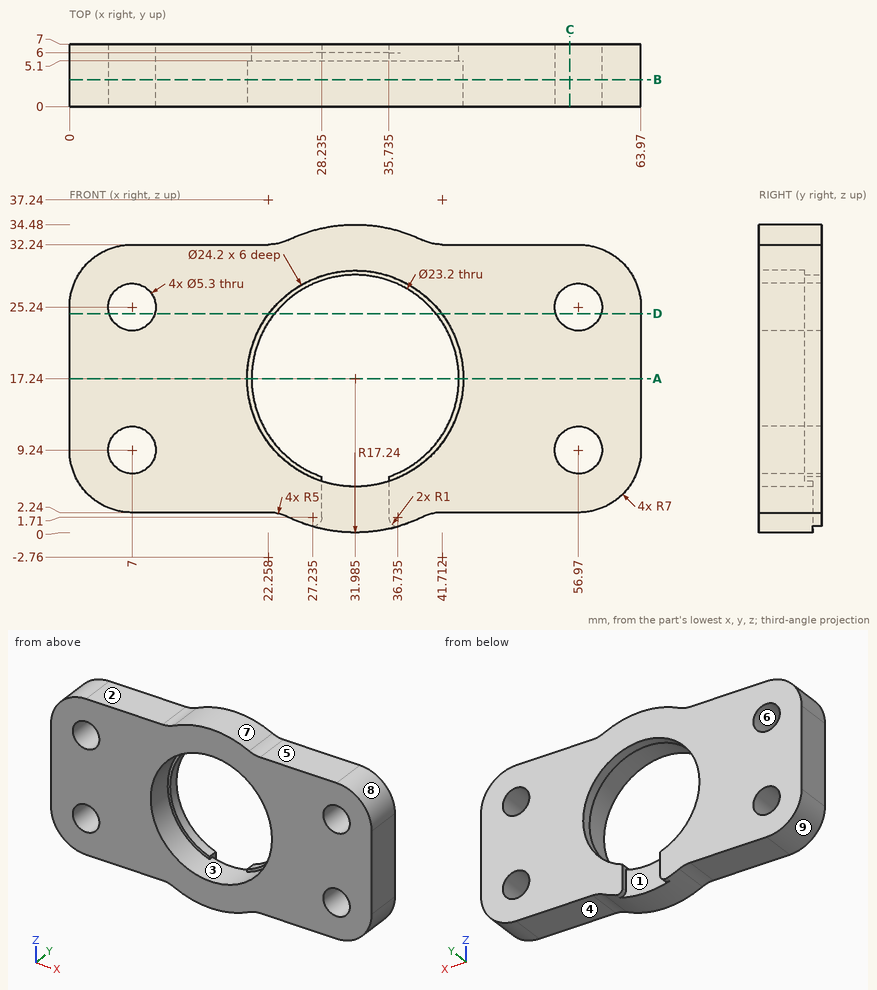
Study the drawing (mm; zero at the part's minimum x, y, z) and answer. A direction names the side the tool comes from. Coordinates: 2 decimals unless noted, no trailing zeros. Write each loop counter-clockwise with the first axis right and the second up, starting at its lowest first coordinate (ties: lowest second). Pieces come first, ordered by that corner, then holes. Notation, with made-up numbers: (33.25, 19) - (64.25, 19) arc R14 cw to (64.25, 40) - close; hole circle Ø6 at (-23.75, -35.5). An arc over 180 degrees is marked (long way). Answer as a JSON object with one key per item and string values.
Q1. For a pull along X with two mould halves and no side action, classify the marked faces 6, 7, 8 and 9 as pulls with the +X half, pulls with the -X half, needs draft (parallel to the pull), parting line crosses it, or undercut.
Results list:
{"face 6": "undercut", "face 7": "parting line crosses it", "face 8": "pulls with the +X half", "face 9": "pulls with the -X half"}
Q2. Consider L1, parallel to Z at x = 55.5, y = 1.5 (1 decimal); L2, parallel to Z at x = 9, y = 3.5; L3, parallel to X at y = 3.5, z = 27.5 (1 decimal). Determine where each line is inside the solid, lowest interval first. Write a range as from..to.
Results list:
{"L1": "z = 2.2..7, 11.4..23, 27.4..32.2", "L2": "z = 2.24..7.5, 10.98..23.5, 26.98..32.24", "L3": "x = 0.4..5.6, 8.4..25.6, 38.4..55.6, 58.4..63.6"}
Q3. Given pin 1 Ø4 at (x, z) = (56.97, 25.24) entering from +Y; pin 2 Ø1.5 at (y, z) = (6, 3.5) entering from -X; pin 3 Ø3 at (y, z) = (3.5, 7.5) entering from +X; pin 4 Ø2 at (x, y) = (17, 3) entering from +Z, each flat-ended and moving along its own axis, determine where each tip first touches the part or whether it passes through.
Results list:
{"pin 1": "passes through", "pin 2": "stops at x = 2.09", "pin 3": "stops at x = 63.97", "pin 4": "stops at z = 32.24"}
Q4. Find section A-A (z = 17.24). Write down the section's boundary in (x, y) (3 decimals).
Results list:
{"outline": "(0, 0) - (19.885, 0) - (19.885, 5.1) - (20.385, 5.1) - (20.385, 7) - (0, 7) - close; (43.585, 5.1) - (44.085, 5.1) - (44.085, 0) - (63.97, 0) - (63.97, 7) - (43.585, 7) - close"}
Q5. Find section B-B (y = 3). State how many separate pieces and enclosed holes the cut face has, plus the area to 3 significant figures.
Results list:
{"separate pieces": "1", "enclosed holes": "5", "area": "1,380 mm^2"}
Q6. Which of the six approach directions +Z, -Z, +X, -X, +Y, -Y give full straight-line access (tool end or side, diameter ignored) to the marked faces 1, 2, 3, 4 and 5?
Results list:
{"face 1": "-Z, +Y", "face 2": "+Z, -X, +Y, -Y", "face 3": "-Y", "face 4": "-Z, +X, +Y, -Y", "face 5": "+Z, +X, +Y, -Y"}
Q7. Find section D-D (z = 24.5). Write down the section's boundary in (x, y) (1 decimal), plus the area to 3 significant figures.
Results list:
{"outline": "(0, 0) - (4.5, 0) - (4.5, 7) - (0, 7) - close; (9.5, 0) - (22.3, 0) - (22.3, 5.1) - (22.9, 5.1) - (22.9, 7) - (9.5, 7) - close; (41, 5.1) - (41.7, 5.1) - (41.7, 0) - (54.4, 0) - (54.4, 7) - (41, 7) - close; (59.5, 0) - (64, 0) - (64, 7) - (59.5, 7) - close", "area": "243 mm^2"}
Q8. Find section C-C (x = 56). Write down the section's boundary in (y, z), plus the area to 3 significant figures.
Results list:
{"outline": "(0, 2.24) - (7, 2.24) - (7, 6.77) - (0, 6.77) - close; (0, 11.71) - (7, 11.71) - (7, 22.77) - (0, 22.77) - close; (0, 27.71) - (7, 27.71) - (7, 32.24) - (0, 32.24) - close", "area": "141 mm^2"}
